Read the model definition and answer for the solid it produces. Units are mm, in the model's axes. Coordinates: 2 decimals unless noted, no trailing zeros. Loops run counter-clockwise (first coordinate to the right, second up) from the corner with the lowest first, then second, coordinate; pieces in that order, holes last. Notation, with made-up numbers: (26, -13.75) -> (53, -13.75) arc R26 cw to (53, 4.25) -> close; hole circle Ø1 at (89.25, 7.5). An arc over 180 degrees is marked (long way). Answer in a Markdown table with one row per item.
Autodesk Inventor part; units mm, degrees
ref_plane "YZ Plane" through (0, 0, 0) normal (1, 0, 0) x (0, 1, 0)
ref_plane "XZ Plane" through (0, 0, 0) normal (0, 1, 0) x (-1, 0, 0)
ref_plane "XY Plane" through (0, 0, 0) normal (0, 0, 1) x (1, 0, 0)
sketch "스케치1" plane through (0, 0, 0) normal (0, 0, 1) x (1, 0, 0)
  line L0 (16.9047, -36.2523) -> (26.8143, -31.6314)
  arc A0 (17.3077, -34.3271) -> (17.3407, -34.809) centre (18.2923, -34.5019) ccw
  line L1 (20, -34.809) -> (17.8869, -30.2774)
  line L2 (20, -34.809) -> (25, -34.809) construction
  line L3 (17.8869, -30.2774) -> (26.834, -26.1053)
  arc A1 (26.8143, -31.6314) -> (26.834, -26.1053) centre (-14.2701, -28.7218) ccw
  line L4 (26.834, -26.1053) -> (17.7607, -30.3363)
  arc A2 (16.9047, -36.2523) -> (17.7607, -30.3363) centre (-14.2701, -28.7218) ccw
  line L5 (26.834, -26.1053) -> (16.9047, -36.2523)
  line L6 (17.9253, -30.3598) -> (26.8143, -31.6314)
  circle A3 centre (22.0881, -30.9553) radius 1.6
  point P0 (0, 0)
  point P1 (12.3536, 2.7038)
  point P2 (0.5383, -0.2738)
  dimension "d0" = 5
  dimension "d1" = 115
  dimension "d2" = 90
  dimension "d3" = 3.2
extrude "돌출1" add sketch "스케치1" along normal blind 56.8
sketch "스케치2" plane through (0, 0, 56.8) normal (0, 0, 1) x (1, 0, 0)
  line L0 (16.9047, -36.2523) -> (26.8143, -31.6314)
  arc A0 (17.3077, -34.3271) -> (18.715, -35.4082) centre (18.2923, -34.5019) ccw
  arc A1 (26.2765, -31.8822) -> (26.8523, -31.032) centre (25.8539, -30.9759) ccw
  line L1 (20, -34.809) -> (17.8869, -30.2774)
  line L2 (20, -34.809) -> (25, -34.809) construction
  line L3 (17.8869, -30.2774) -> (26.834, -26.1053)
  arc A2 (26.8143, -31.6314) -> (12, 3) centre (-14.2701, -28.7218) ccw
  line L4 (26.834, -26.1053) -> (17.7607, -30.3363)
  arc A3 (16.9047, -36.2523) -> (0, 0) centre (-14.2701, -28.7218) ccw
  arc A4 (26.2765, -31.8822) -> (26.8523, -31.032) centre (25.8539, -30.9759) ccw
  circle A5 centre (22.0881, -30.9553) radius 1.6
  line L5 (26.834, -26.1053) -> (22.0881, -30.9553)
  line L6 (19.4569, -33.6442) -> (16.9047, -36.2523)
  line L7 (17.7607, -30.3363) -> (20.5042, -30.7287)
  line L8 (23.6719, -31.1819) -> (26.8143, -31.6314)
  point P0 (12.3536, 2.7038)
  point P1 (0.5383, -0.2738)
  dimension "d6" = 5
  dimension "d7" = 115
  dimension "d8" = 90
  dimension "d9" = 3.2
extrude "돌출2" cut sketch "스케치2" against normal up to surface (56.8 mm away) contours A5
sketch "스케치3" plane through (26.8143, -31.6314, 0) normal (0.4226183, -0.9063078, 0) x (0.9063078, 0.4226183, 0)
  line L0 (-10.934, -4.1) -> (0, -4.1)
  line L1 (0, -4.1) -> (0, 60.9)
  line L2 (0, 60.9) -> (-10.934, 60.9)
  line L3 (-10.934, 60.9) -> (-10.934, -4.1)
  line L4 (0, 0) -> (0, 56.8)
  line L5 (-10.934, 0) -> (-10.934, 56.8)
  dimension "d12" = 65
  dimension "d13" = 4.1
  dimension "d14" = 10.934
  dimension "d15" = 10.934
  dimension "d16" = 10.934
extrude "돌출3" add sketch "스케치3" along normal blind 3
sketch "스케치4" plane through (0, 0, 0) normal (0, 0, -1) x (-1, 0, 0)
  circle A0 centre (-6, 44) radius 4.8
  circle A1 centre (-6, 9) radius 4.8
  circle A2 centre (-9.8616, -1.4411) radius 1.6
  circle A3 centre (-22.0881, -30.9553) radius 1.6
  arc A4 (0, 44) -> (-12, 44) centre (-6, 44) ccw
  line L0 (-12, 6.562) -> (-12, 44)
  arc A5 (-14.4262, 0.8233) -> (-12, 6.562) centre (-20, 6.562) ccw
  arc A6 (-14.4262, 0.8233) -> (-26.8143, -31.6314) centre (14.2701, -28.7218) ccw
  line L1 (-16.9047, -36.2523) -> (-26.8143, -31.6314)
  line L2 (-16.9047, -36.2523) -> (0, 0)
  line L3 (0, 44) -> (0, 0)
  line L4 (-16.9047, -36.2523) -> (-26.8143, -31.6314)
  line L5 (-26.8143, -31.6314) -> (-28.0821, -34.3503)
  line L6 (-18.1726, -38.9712) -> (-28.0821, -34.3503)
  line L7 (-16.9047, -36.2523) -> (-18.1726, -38.9712)
  circle A7 centre (-22.0881, -30.9553) radius 1.6
  line L8 (-16.9047, -36.2523) -> (-26.8143, -31.6314)
  arc A8 (-17.7607, -30.3363) -> (-16.9047, -36.2523) centre (14.2701, -28.7218) ccw
  line L9 (-26.834, -26.1053) -> (-17.7607, -30.3363)
  arc A9 (-26.834, -26.1053) -> (-26.8143, -31.6314) centre (14.2701, -28.7218) ccw
  line L10 (-16.9047, -36.2523) -> (-26.8143, -31.6314)
  line L11 (-21.8595, -33.9419) -> (-5.8, 0.4978) construction
  line L12 (-5.8, 0.4978) -> (-0.8452, -1.8126)
  line L13 (-5.8, 0.4978) -> (-12.5505, 3.6456)
  point P0 (0, 0)
  point P1 (0, 0)
  point P2 (-17.7151, -2.7731)
  dimension "d19" = 38
extrude "돌출4" add sketch "스케치4" against normal up to surface (56.8 mm away) contours L2 A8 L9 A6 A5 L13 L12
sketch "스케치8" plane through (16.9047, -36.2523, -4.1) normal (-0.9063078, -0.4226183, 0) x (0, 0, 1)
  line L0 (4.1, 38) -> (60.9, 38)
  line L1 (4.1, 0) -> (4.1, 38)
  line L2 (65, 0) -> (60.9, 0)
  line L3 (0, 0) -> (0, -3)
  line L4 (65, -3) -> (0, -3)
  line L5 (65, 0) -> (65, -3)
  line L6 (4.1, 0) -> (0, 0)
  line L7 (60.9, 0) -> (60.9, 38)
  line L8 (4.1, 0) -> (4.1, 34.6494)
  line L9 (61.1, 38) -> (4.1, 38)
  line L10 (4.1, 38) -> (4.1, 0)
  line L11 (4.1, 0) -> (61.1, 0)
  line L12 (61.1, 0) -> (61.1, 38)
  line L13 (4.1, 38) -> (61.1, 38)
  line L14 (32.6, 38) -> (32.6, 19)
  line L15 (60.9, 0) -> (60.9, 38)
  line L16 (60.9, 19.0005) -> (4.1, 19)
  line L17 (57.6, 34) -> (7.6, 34)
  line L18 (7.6, 34) -> (7.6, 4)
  line L19 (7.6, 4) -> (57.6, 4)
  line L20 (57.6, 4) -> (57.6, 34)
  line L21 (57.6, 34) -> (7.6, 4) construction
  line L22 (7.6, 34) -> (57.6, 4) construction
  point P0 (4.1, 40)
  dimension "d37" = 50
  dimension "d38" = 30
extrude "돌출7" cut sketch "스케치8" against normal blind 3 contours L17 L20 L16 L14 | L14 L16 L18 L17 | L16 L20 L19 L18
equation "\"d15\" = d14"
equation "\"d16\" = d14"
properties part number "Grip_Side_Down" material "LCP 플라스틱"
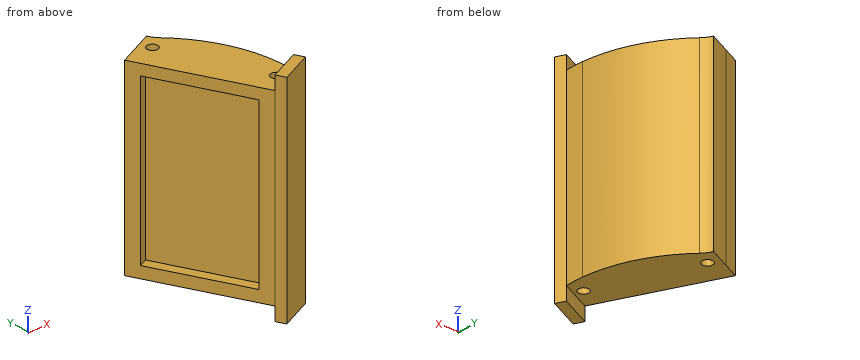
1. A cutting plane is placed at A-A on x = 21.5. Give the vertices of the cut face in (y, z), and give its area (3 significant figures).
A:
| item | result |
|---|---|
| outline | (-37.42, -4.1) -> (-34.11, -4.1) -> (-34.11, 0) -> (-32.44, 0) -> (-32.44, 56.8) -> (-34.11, 56.8) -> (-34.11, 60.9) -> (-37.42, 60.9) -> close; (-29.47, 0) -> (-8.3, 0) -> (-8.3, 56.8) -> (-29.47, 56.8) -> close |
| area | 1,510 mm2 |
2. A cutting plane is placed at C-C on z = 13. Give the vertices of the cut face in (x, y), and give its area (3 significant figures).
A:
| item | result |
|---|---|
| outline | (0.85, -1.81) -> (2.54, -5.44) -> (5.26, -4.17) -> (17.93, -31.36) -> (15.21, -32.63) -> (16.9, -36.25) -> (18.17, -38.97) -> (28.08, -34.35) -> (26.81, -31.63) arc R41.19 ccw to (26.83, -26.11) arc R41.19 ccw to (14.43, 0.82) arc R8 cw to (12.55, 3.65) -> (5.8, 0.5) -> close; hole circle Ø3.2 at (9.86, -1.44); hole circle Ø3.2 at (22.09, -30.96) |
| area | 482 mm2 |
3. A cutting plane is placed at D-D on x = 6.5. Give the vertices of the cut face in (y, z).
A:
| item | result |
|---|---|
| outline | (-13.94, 0) -> (0.82, 0) -> (0.82, 56.8) -> (-13.94, 56.8) -> (-13.94, 53.5) -> (-6.84, 53.5) -> (-6.84, 3.5) -> (-13.94, 3.5) -> close |
4. A cutting plane is placed at B-B on y = -27. Give the vertices of the cut face in (x, z).
A:
| item | result |
|---|---|
| outline | (12.59, 0) -> (26.88, 0) -> (26.88, 56.8) -> (12.59, 56.8) -> (12.59, 53.5) -> (15.9, 53.5) -> (15.9, 3.5) -> (12.59, 3.5) -> close |
5. Find the intervals of material crossed by probe 1 along Z at (x, y) = (10, -18); probe 2 along Z at (x, y) = (10, -13.5); probe 3 along Y at (x, z) = (21.75, 2), in increasing order.
A:
| item | result |
|---|---|
| probe 1 | z = 0 to 3.5, 53.5 to 56.8 |
| probe 2 | z = 0 to 56.8 |
| probe 3 | y = -37.3 to -32.52, -29.39 to -8.75 |
6. Given pin 1 Ø1 at (x, y) = (21.5, -14.5) entering from -Z; pin 2 Ø10 at (x, y) = (19.5, -14) entering from +Z; pin 3 Ø1 at (y, z) = (-9, 46) entering from -X, each flat-ended and moving along its own axis, determine where each tip first touches the part or whether it passes through.
A:
| item | result |
|---|---|
| pin 1 | stops at z = 0 |
| pin 2 | stops at z = 56.8 |
| pin 3 | stops at x = 7.28 |
